from build123d import *

# Parameters (mm, degrees)
SKETCH1_R           = 10
BOSS_EXTRUDE1_DEPTH = 22
CUT_EXTRUDE1_DEPTH  = 12
CUT_EXTRUDE2_DEPTH  = 10
SKETCH5_W           = 16
SKETCH5_H           = 4
CUT_EXTRUDE4_DEPTH  = 23
SKETCH4_R           = 1.5
CUT_EXTRUDE3_DEPTH  = 13


with BuildPart() as part:
    # Sketch1 → Boss-Extrude1 (new body)
    with BuildSketch(Plane(origin=(0, 0, 0), x_dir=(0, 0, -1), z_dir=(1, 0, 0))):
        Circle(SKETCH1_R)
    extrude(amount=BOSS_EXTRUDE1_DEPTH)

    # Sketch2 → Cut-Extrude1 (cut)
    with BuildSketch(Plane.ZY):
        with BuildLine():
            Line((-2, 3.464101615), (2, 3.464101615))
            ThreePointArc((2, 3.464101615), (0, -4), (-2, 3.464101615))
        make_face()
    extrude(amount=-CUT_EXTRUDE1_DEPTH, mode=Mode.SUBTRACT)

    # Sketch3 → Cut-Extrude2 (cut)
    with BuildSketch(Plane(origin=(22, 0, 0), x_dir=(0, 0, -1), z_dir=(1, 0, 0))):
        with BuildLine():
            Line((-2.449489743, 0.5), (-9.987492178, 0.5))
            ThreePointArc((-9.987492178, 0.5), (-9.996872555, 0.250078211), (-10, 0))
            ThreePointArc((-10, 0), (-9.996872555, -0.250078211), (-9.987492178, -0.5))
            Line((-9.987492178, -0.5), (-2.449489743, -0.5))
            ThreePointArc((-2.449489743, -0.5), (-2.5, 0), (-2.449489743, 0.5))
        make_face()
        with BuildLine():
            ThreePointArc((10, 0), (9.996872555, 0.250078211), (9.987492178, 0.5))
            Line((9.987492178, 0.5), (2.449489743, 0.5))
            ThreePointArc((2.449489743, 0.5), (2.487340383, 0.251272405), (2.5, 0))
            ThreePointArc((2.5, 0), (2.487340383, -0.251272405), (2.449489743, -0.5))
            Line((2.449489743, -0.5), (9.987492178, -0.5))
            ThreePointArc((9.987492178, -0.5), (9.996872555, -0.250078211), (10, 0))
        make_face()
        with BuildLine():
            Line((2.449489743, -0.5), (-2.449489743, -0.5))
            ThreePointArc((-2.449489743, -0.5), (0, -2.5), (2.449489743, -0.5))
        make_face()
        with BuildLine():
            Line((2.449489743, 0.5), (-2.449489743, 0.5))
            ThreePointArc((-2.449489743, 0.5), (-2.5, 0), (-2.449489743, -0.5))
            Line((-2.449489743, -0.5), (2.449489743, -0.5))
            ThreePointArc((2.449489743, -0.5), (2.487340383, -0.251272405), (2.5, 0))
            ThreePointArc((2.5, 0), (2.487340383, 0.251272405), (2.449489743, 0.5))
        make_face()
        with BuildLine():
            ThreePointArc((2.449489743, 0.5), (0, 2.5), (-2.449489743, 0.5))
            Line((-2.449489743, 0.5), (2.449489743, 0.5))
        make_face()
    extrude(amount=-CUT_EXTRUDE2_DEPTH, mode=Mode.SUBTRACT)

    # Sketch5 → Cut-Extrude4 (cut, through all)
    with BuildSketch(Plane(origin=(22, 0, 0), x_dir=(0, 0, -1), z_dir=(1, 0, 0))):
        with Locations((0, 8)):
            Rectangle(SKETCH5_W, SKETCH5_H)
        with Locations((0, -8)):
            Rectangle(SKETCH5_W, SKETCH5_H)
    extrude(amount=-CUT_EXTRUDE4_DEPTH, mode=Mode.SUBTRACT)

    # Sketch4 → Cut-Extrude3 (cut, through all)
    with BuildSketch(Plane(origin=(0, 6, 0), x_dir=(1, 0, 0), z_dir=(0, 1, 0))):
        with Locations((18, 5.5)):
            Circle(SKETCH4_R)
        with Locations((18, -5.5)):
            Circle(SKETCH4_R)
    extrude(amount=-CUT_EXTRUDE3_DEPTH, mode=Mode.SUBTRACT)


solid = part.part
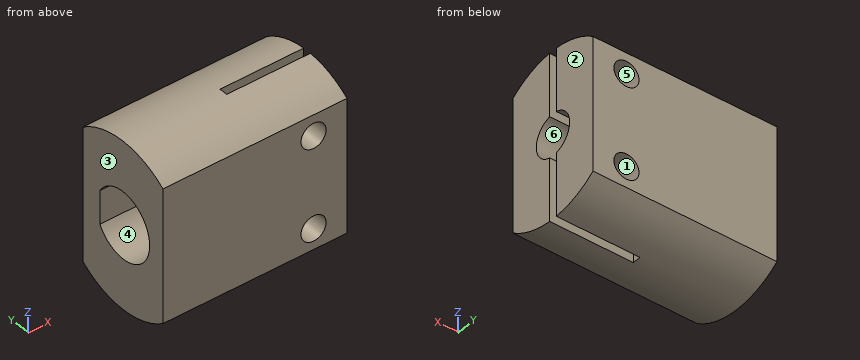
Model file for the job. Use its own axes, mm. Face numbers are marked on the shaded views. A direction names the side the tool comes from. Coordinates: 2 decimals unless noted, no trailing zeros. Order: outer loops, then holes, each group sorted by start corner. A loop starts at its lowest first (then second) coordinate and runs counter-clockwise, first axis right, second up. Notation, with made-up numbers: (-19, 47.25) -> (-9, 47.25) arc R19 ccw to (-9, 63.25) -> close; hole circle Ø8 at (46.5, 15). An arc over 180 degrees is marked (long way). Return JSON: item names as keys, results as strings. Group by question number.
Item 1: Flat gauge pins, fed straight in: P1, Ø3, axis at y = -1.5, z = 0, coming from the -X side; P2, Ø0.8, axis at y = 0, z = 8.5, coming from the +X side; P3, Ø1.8, axis at x = 18, z = -5.5, coming from the +Y side; P4, Ø5, axis at x = 18, z = -5.5, coming from the +Y side. Where does each tip first touch, or does it go through?
Item 2: Wall check: line 1 along Y through (x, z) = (13, -0.5); line 2 along Y through (x, z) = (15.25, 4.75); line 3 along X through (y, z) = (-2.8, 5.5). Give the ranges that are in metal, low to high. Write a range as [from, to].
Item 3: Saw through at C-C on y = 0. Write the cut outline in (x, z).
Item 4: Saw through at D-D on x = 13. Write the cut outline in (y, z).
Item 5: Saw through at A-A on z = 0.5. Write the cut outline in (x, y), then the cut area to 3 significant figures.
Item 6: Saw through at B-B on x = 18. Write the cut outline in (y, z).
Item 7: Pull direction X, two halves, no side cores. Call the marked faces 1, 2 and 3: pulls with the +X half, pulls with the -X half, needs draft (parallel to the pull), parting line crosses it, or undercut.
Item 8: Tool access for the marked faces 4, 5 and 6: list every direction of +Z, -Z, +X, -X, +Y, -Y with a clear straight run to the whole face (end or side of a thin tool).
Values found:
{
 "1": {"P1": "stops at x = 12", "P2": "stops at x = 12", "P3": "passes through", "P4": "stops at y = 6"},
 "2": {"line 1": "y = [-6, -2.45], [2.45, 6]", "line 2": "y = [-6, -0.5], [0.5, 6]", "line 3": "x = [0, 16.5], [19.5, 22]"},
 "3": {"outline": "(0, -10) -> (12, -10) -> (12, -4) -> (0, -4) -> close; (0, 4) -> (12, 4) -> (12, 10) -> (0, 10) -> close"},
 "4": {"outline": "(-6, -8) arc R10 ccw to (-0.5, -9.99) -> (-0.5, -2.45) arc R2.5 cw to (-0.5, 2.45) -> (-0.5, 9.99) arc R10 ccw to (-6, 8) -> close; (0.5, -9.99) arc R10 ccw to (6, -8) -> (6, 8) arc R10 ccw to (0.5, 9.99) -> (0.5, 2.45) arc R2.5 cw to (0.5, -2.45) -> close"},
 "5": {"outline": "(0, -6) -> (22, -6) -> (22, -2.45) -> (12, -2.45) -> (12, -3.97) -> (0, -3.97) -> close; (0, 3.46) -> (12, 3.46) -> (12, 2.45) -> (22, 2.45) -> (22, 6) -> (0, 6) -> close", "area": "126 mm2"},
 "6": {"outline": "(-6, -8) arc R10 ccw to (-0.5, -9.99) -> (-0.5, -7) -> (-6, -7) -> close; (-6, -4) -> (-0.5, -4) -> (-0.5, -2.45) arc R2.5 cw to (-0.5, 2.45) -> (-0.5, 4) -> (-6, 4) -> close; (-6, 7) -> (-0.5, 7) -> (-0.5, 9.99) arc R10 ccw to (-6, 8) -> close; (0.5, -9.99) arc R10 ccw to (6, -8) -> (6, -7) -> (0.5, -7) -> close; (0.5, -4) -> (6, -4) -> (6, 4) -> (0.5, 4) -> (0.5, 2.45) arc R2.5 cw to (0.5, -2.45) -> close; (0.5, 7) -> (6, 7) -> (6, 8) arc R10 ccw to (0.5, 9.99) -> close"},
 "7": {"face 1": "undercut", "face 2": "pulls with the +X half", "face 3": "pulls with the -X half"},
 "8": {"face 4": "-X", "face 5": "+Y, -Y", "face 6": "+X, -X"}
}
